Input: dimensioned drawing with shaded views. Units: mm. Origin: part minimum x, y, z. A direction names the side the tool comes from. Round coordinates to 2 decimals unless told otherwise and drop trailing zeros. Order: outer loops, then holes, each group sorted by start corner. A loop starts at its lowest first (then second) coordinate and runs counter-clockwise, first axis right, second up. Notation, with made-up numbers: (-21.5, 89) -> (16.5, 89) arc R22 cw to (16.5, 125) -> close; hole circle Ø9 at (71.5, 12.25). An arc over 180 degrees is marked (long way). Use a Markdown table: item, result. Add a question column.
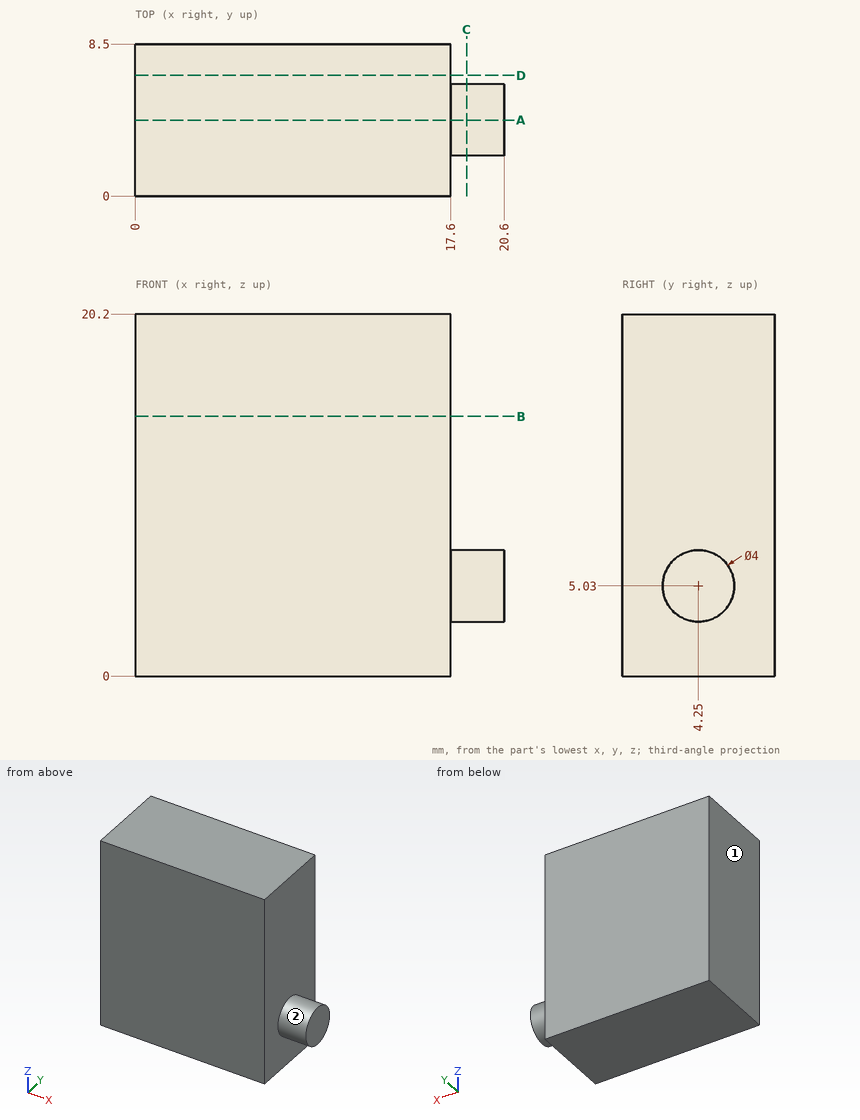
1) Line query: probe 1 along X at (y, z) = (6.5, 19); probe 2 along Z at (x, y) = (19.75, 3). Output: solid intervals per line, ascending. Write a range as from..to.
2) Section B-B on z = 14.5. Output: boundary loops of the cut face in (x, y), then the cut area to 3 significant figures.
3) First-contact query: pin 1 Ø2.5 at (y, z) = (3, 15) entering from +X. Flat tip, straight axial feed; report the tip coordinate or a pass-through.
4) Section C-C on x = 18.5. Output: boundary loops of the cut face in (y, z), then the cut area to 3 significant figures.
5) Reachability of the marked faces 1 and 2 from +Z, -Z, +X, -X, +Y, -Y: full face, straight path, thin tool, end or side. Return the list, or none.
6) Section D-D on y = 6.75. Output: boundary loops of the cut face in (x, z), then the cut area to 3 significant figures.
7) Section A-A on y = 4.25. Output: boundary loops of the cut face in (x, z).
Conclusion:
| question | item | result |
|---|---|---|
| 1 | probe 1 | x = 0..17.6 |
| 1 | probe 2 | z = 3.47..6.59 |
| 2 | outline | (0, 0) -> (17.6, 0) -> (17.6, 8.5) -> (0, 8.5) -> close |
| 2 | area | 150 mm^2 |
| 3 | pin 1 | stops at x = 17.6 |
| 4 | outline | circle Ø4 at (4.25, 5.03) |
| 4 | area | 12.6 mm^2 |
| 5 | face 1 | +Z, -Z, -X, +Y, -Y |
| 5 | face 2 | +X |
| 6 | outline | (0, 0) -> (17.6, 0) -> (17.6, 20.2) -> (0, 20.2) -> close |
| 6 | area | 356 mm^2 |
| 7 | outline | (0, 0) -> (17.6, 0) -> (17.6, 3.03) -> (20.6, 3.03) -> (20.6, 7.03) -> (17.6, 7.03) -> (17.6, 20.2) -> (0, 20.2) -> close |
